Read the model definition and answer for the solid it produces. Units are mm, in the model's axes. A direction names the side the tool comes from. Round coordinates to 2 decimals unless told otherwise and drop trailing zeros. Write each loop counter-clockwise with the first axis right and the second up, starting at its lowest first coordinate (ties: lowest second). Pieces come first, ordered by that corner, then holes. Notation, with made-up numbers: (25, 78.25) -> (47, 78.25) arc R33 cw to (47, 116.25) -> close; hole circle Ø1 at (11.25, 71.25). An arc over 180 degrees is marked (long way). Return JSON: item names as keys, results as strings.
Autodesk Inventor part; units mm, degrees
ref_plane "YZ Plane" through (0, 0, 0) normal (1, 0, 0) x (0, 1, 0)
ref_plane "XZ Plane" through (0, 0, 0) normal (0, 1, 0) x (-1, 0, 0)
ref_plane "XY Plane" through (0, 0, 0) normal (0, 0, 1) x (1, 0, 0)
sketch "Sketch1" plane through (0, 0, 0) normal (0, 1, 0) x (-1, 0, 0)
  line L0 (10, 10.5) -> (-10, 10.5)
  line L1 (-10, 10.5) -> (-10, -10.5)
  line L2 (-10, -10.5) -> (10, -10.5)
  line L3 (10, -10.5) -> (10, 10.5)
  line L4 (10, 10.5) -> (-10, -10.5) construction
  line L5 (-10, 10.5) -> (10, -10.5) construction
  line L6 (8, 8.5) -> (-8, 8.5)
  line L7 (-8, 8.5) -> (-8, -8.5)
  line L8 (-8, -8.5) -> (8, -8.5)
  line L9 (8, -8.5) -> (8, 8.5)
  point P0 (0, 0)
  dimension "d0" = 20
  dimension "d1" = 21
  dimension "d2" = 2
extrude "Extrusion1" add sketch "Sketch1" against normal blind 1.5 contours L3 L2 L1 L0 | L9 L8 L7 L6
hole "Hole1" at (-8, 0, 8.5) at (-8, 0, -8.5) at (8, 0, -8.5) at (8, 0, 8.5) direction (0, -1, 0) diameter 2 end through all
sketch "Sketch2" plane through (0, 0, 0) normal (0, 1, 0) x (1, 0, 0)
  line L0 (-3.85, -8.5124) -> (3.85, -8.5124)
  line L1 (3.85, -8.5124) -> (3.85, -17.5124)
  line L2 (3.85, -17.5124) -> (-3.85, -17.5124)
  line L3 (-3.85, -17.5124) -> (-3.85, -8.5124)
  line L4 (-3.85, -8.5124) -> (3.85, -17.5124) construction
  line L5 (3.85, -8.5124) -> (-3.85, -17.5124) construction
  line L6 (-10, -10.5) -> (10, -10.5)
  line L7 (-10, 10.5) -> (-10, -10.5)
  point P0 (0, 0)
  point P1 (0, -13.0124)
  point P2 (0, -8.5124)
  point P3 (0, -8.5124)
  dimension "d12" = 7.7
  dimension "d13" = 9
  dimension "d14" = 1.9876
  dimension "d15" = 10
extrude "Extrusion2" add sketch "Sketch2" along normal blind 4
sketch "Sketch3" plane through (0, 0, 0) normal (0, 1, 0) x (1, 0, 0)
  circle A0 centre (0, 0) radius 5.85
  dimension "d18" = 11.7
extrude "Extrusion3" add sketch "Sketch3" along normal blind 9
properties part number "buzzer_footprint"
Item 1: Section C-C (y = 3) is taken. Give the vertices of the cut face in (x, z), then the cut area to 3 significant figures.
Worked answers:
{"outline": "circle Ø11.7 at (0, 0); (-3.85, 8.51) -> (3.85, 8.51) -> (3.85, 17.51) -> (-3.85, 17.51) -> close", "area": "177 mm2"}
Item 2: Section B-B (z = -8.5) is taken. Give the vertices of the cut face in (x, y), then the cut area to 3 significant figures.
Worked answers:
{"outline": "(-10, -1.5) -> (-9, -1.5) -> (-9, 0) -> (-10, 0) -> close; (-7, -1.5) -> (7, -1.5) -> (7, 0) -> (-7, 0) -> close; (9, -1.5) -> (10, -1.5) -> (10, 0) -> (9, 0) -> close", "area": "24.0 mm2"}
Item 3: Section A-A (x = 8) is taken. Give the vertices of the cut face in (y, z).
Worked answers:
{"outline": "(-1.5, -10.5) -> (0, -10.5) -> (0, -9.5) -> (-1.5, -9.5) -> close; (-1.5, -7.5) -> (0, -7.5) -> (0, 7.5) -> (-1.5, 7.5) -> close; (-1.5, 9.5) -> (0, 9.5) -> (0, 10.5) -> (-1.5, 10.5) -> close"}
Item 4: A tool of negligible diameter and unlimited length cuts with its end or side. For faces 1 (the flat face through (0, 0, 14)), 2 (the cylindrical face through (-1.27, 4.44, -5.71)), 3 (the flat face through (0, 2, 8.512)), from which of +Z, -Z, +X, -X, +Y, -Y can it reach the whole face along a straight path? Write none if from no direction.
Worked answers:
{"face 1": "+Z, +X, -X, -Y", "face 2": "+Y", "face 3": "+X, -X, +Y"}
Item 5: Straight lines are drawn through the part: L1, parallel to X at y = -0.8, z = 8.5; L2, parallel to Z at x = 8, y = -0.45; L3, parallel to Y at x = -6.5, z = -0.5. For each, find the intervals that lie inside material, in ascending order. Write a range as [from, to].
Worked answers:
{"L1": "x = [-10, -9], [-7, 7], [9, 10]", "L2": "z = [-10.5, -9.5], [-7.5, 7.5], [9.5, 10.5]", "L3": "y = [-1.5, 0]"}
Item 6: For a pull along Z with two mould halves and no side action, classify faces 4 (the flat face through (0, 2, 17.512)), 5 (the flat face through (0, -1.5, 0)), 6 (the cylindrical face through (7.01, -0.76, 8.37)) as released by +Z, released by -Z, zero draft, split by the parting line, or undercut.
Worked answers:
{"face 4": "released by +Z", "face 5": "zero draft", "face 6": "undercut"}
Item 7: Section D-D (z = 0) is taken. Give the vertices of the cut face in (x, y).
Worked answers:
{"outline": "(-10, -1.5) -> (10, -1.5) -> (10, 0) -> (5.85, 0) -> (5.85, 9) -> (-5.85, 9) -> (-5.85, 0) -> (-10, 0) -> close"}
Item 8: Flat-ended cylindrical pins translate along their axes: pin 1 (4 mm diameter, centred on y = 4, z = 5, fed in from -X); pin 2 (1.5 mm diameter, centred on x = -2, y = 3, fed in from -Z); pin 3 (1.2 mm diameter, centred on y = 2, z = 13.5, fed in from +X). Find the tip coordinate at first contact, or state that the pin passes through.
Worked answers:
{"pin 1": "stops at x = -5.02", "pin 2": "stops at z = -5.71", "pin 3": "stops at x = 3.85"}
